Source: CAD feature listing. Evaluate the final solid. Frame: model axes, mm. Coordinates: 2 decimals unless noted, no trailing zeros. Loops run counter-clockwise (first coordinate to the right, second up) from the corner with the lowest first, then second, coordinate; pieces in that order, holes last. Notation, with made-up numbers: (70.5, 77) - (97.5, 77) arc R21 ccw to (97.5, 91) - close; hole circle Ø6 at (-37, -2). An arc over 180 degrees is marked (long way). Use one line per item in the form item = value. Start each with the question number.
from build123d import *

# Parameters (mm, degrees)
F0_W     = 39.190798
F0_H     = 12.7
F0_W_2   = 212.120296
F3_W     = 5.08
F3_H     = 13.252163
F3_W_2   = 19.028907
F3_H_2   = 5.08
F4_DEPTH = 2.54
F5_DEPTH = 2.54


with BuildPart() as f1:
    # F0 (on Front) → F1 (revolve)
    with BuildSketch(Plane.XZ):
        with Locations((19.595399, 6.35)):
            Rectangle(F0_W, F0_H)
        with Locations((145.250946, 6.35)):
            Rectangle(F0_W_2, F0_H)
        Polygon((279.4, 12.7), (251.311094, 12.7), (251.311094, 0), (276.86, 0), (276.86, 6.35), (279.4, 6.35), align=None)
    revolve(axis=Axis((146.856308, 0, 0), (1, 0, 0)))

    # F3 (on face) → F4 (cut)
    with BuildSketch(Plane.YZ.offset(279.4)):
        with Locations((0, -9.166081)):
            Rectangle(F3_W, F3_H)
        with Locations((12.054453, 0)):
            Rectangle(F3_W_2, F3_H_2)
        with Locations((-12.054453, 0)):
            Rectangle(F3_W_2, F3_H_2)
        with Locations((0, 9.166081)):
            Rectangle(F3_W, F3_H)
    extrude(amount=-F4_DEPTH, mode=Mode.SUBTRACT)

    # F3 (on face) → F5 (cut)
    with BuildSketch(Plane.YZ.offset(279.4)):
        with Locations((0, -9.166081)):
            Rectangle(F3_W, F3_H)
        with Locations((12.054453, 0)):
            Rectangle(F3_W_2, F3_H_2)
        with Locations((-12.054453, 0)):
            Rectangle(F3_W_2, F3_H_2)
        with Locations((0, 9.166081)):
            Rectangle(F3_W, F3_H)
    extrude(amount=-F5_DEPTH, mode=Mode.SUBTRACT)


solid = f1.part
(1) Material intervals for line 1 (Y direction, x = 154, z = 2.5); line 2 (X direction, y = 0.25, z = -4.25), sorted ascending.
(2) Cut plane A-A, the plane z = 10. Output: boundary loops of the cut face in (x, y).
(3) Cut plane C-C, the plane y = 8.25. Output: boundary loops of the cut face in (x, z).
(4) Mould query, pull axis Y, two halves, no side actions, for faces 1 (the face through (279.4, 6, -6)), 2 (the face through (276.86, 1, 0)), 3 (the face through (137.74, 12.4, -2.75)). Classes: +Y half, -Y half, draft (parallel to the pull), parting line (faces both ways), or undercut.
(5) Cut plane B-B, the plane x = 112.5. Output: boundary loops of the cut face in (y, z), plus the area to 3 significant figures.
(6) Contact query for flat-ended pins moving along their axis: pin 1 (1.3 mm diameter, centred on x = 278, y = -8, fed in from -Z); pin 2 (0.8 mm diameter, centred on x = 278, z = 8, fed in from +Y); pin 3 (10 mm diameter, centred on x = 247.5, y = -1, fed in from +Z); pin 4 (2 mm diameter, centred on x = 277.5, z = -9.5, fed in from -Y). Output: stop coordinate, or through.
Recorded:
q1.line_1 = -12.45 to 12.45
q1.line_2 = 0 to 276.86
q2.outline = (0, -7.83) - (279.4, -7.83) - (279.4, -2.54) - (276.86, -2.54) - (276.86, 2.54) - (279.4, 2.54) - (279.4, 7.83) - (0, 7.83) - close
q3.outline = (0, -9.66) - (279.4, -9.66) - (279.4, -2.54) - (276.86, -2.54) - (276.86, 2.54) - (279.4, 2.54) - (279.4, 9.66) - (0, 9.66) - close
q4.face_1 = draft
q4.face_2 = undercut
q4.face_3 = parting line
q5.outline = circle Ø25.4 at (0, 0)
q5.area = 507 mm²
q6.pin_1 = -10.36
q6.pin_2 = 10.17
q6.pin_3 = 12.7
q6.pin_4 = -9.44
